```python
from build123d import *

# Parameters (mm, degrees)
SKETCH1_W           = 53.975
SKETCH1_H           = 31.75
BOSS_EXTRUDE1_DEPTH = 76.2
SHELL1_T            = 5
SKETCH2_W           = 44.45
SKETCH2_H           = 53.975
CUT_EXTRUDE1_DEPTH  = 5
FILLET1_R           = 31.75
FILLET2_R           = 6.35
FILLET3_R           = 6.35
SKETCH3_W           = 44.45
SKETCH3_H           = 53.975
BOSS_EXTRUDE2_DEPTH = 19.05
FILLET5_R           = 3.175
FILLET6_R           = 3.175


with BuildPart() as part:
    # Sketch1 → Boss-Extrude1 (new body)
    with BuildSketch(Plane(origin=(0, 0, 0), x_dir=(0, 0, -1), z_dir=(1, 0, 0))):
        with Locations((106.854663617, 0)):
            Rectangle(SKETCH1_W, SKETCH1_H)
    extrude(amount=BOSS_EXTRUDE1_DEPTH)

    # Shell1
    shell1_openings = [part.faces().sort_by_distance(p)[0] for p in [
        (0, 0, -106.854663617),
    ]]
    offset(amount=SHELL1_T, openings=shell1_openings, kind=Kind.INTERSECTION)

    # Sketch2 → Cut-Extrude1 (cut)
    with BuildSketch(Plane(origin=(0, -20.875, 0), x_dir=(-1, 0, 0), z_dir=(0, -1, 0))):
        with Locations((-53.975, 106.854663617)):
            Rectangle(SKETCH2_W, SKETCH2_H)
    extrude(amount=-CUT_EXTRUDE1_DEPTH, mode=Mode.SUBTRACT)

    # Fillet1
    fillet1_edges = [part.edges().sort_by_distance(p)[0] for p in [
        (76.2, 15.875, -106.854663617),
    ]]
    fillet(fillet1_edges, radius=FILLET1_R)

    # Fillet2
    # the kernel refuses this fillet: 6.35 mm, written as the material it takes off along each edge
    with BuildSketch(Plane(origin=(31.75, -15.875, -79.867163617), x_dir=(-1, 0, 0), z_dir=(0, 0, -1))) as fillet2_piece_1:
        with BuildLine():
            CenterArc((6.204836823, -6.35), FILLET2_R, 90, 77.725329785)
            Line((0, -5), (0, 0))
            Line((0, 0), (6.204836823, 0))
        make_face()
    extrude(amount=53.975, mode=Mode.SUBTRACT)

    # Fillet3
    fillet3_edges = [part.edges().sort_by_distance(p)[0] for p in [
        (81.2, 0, -138.842163617),
        (81.2, 20.875, -106.854663617),
        (81.2, 0, -74.867163617),
        (40.6, 20.875, -74.867163617),
        (40.6, 20.875, -138.842163617),
    ]]
    fillet(fillet3_edges, radius=FILLET3_R)

    # Sketch3 → Boss-Extrude2 (add)
    with BuildSketch(Plane.XZ.offset(20.875)):
        with BuildLine():
            Line((26.67, -74.867163617), (26.67, -138.842163617))
            Line((26.67, -138.842163617), (74.85, -138.842163617))
            ThreePointArc((74.85, -138.842163617), (79.340128061, -136.982291678), (81.2, -132.492163617))
            Line((81.2, -132.492163617), (81.2, -81.217163617))
            ThreePointArc((81.2, -81.217163617), (79.340128061, -76.727035557), (74.85, -74.867163617))
            Line((74.85, -74.867163617), (26.67, -74.867163617))
        make_face()
        with Locations((53.975, -106.854663617)):
            Rectangle(SKETCH3_W, SKETCH3_H, mode=Mode.SUBTRACT)
    extrude(amount=BOSS_EXTRUDE2_DEPTH)

    # Fillet5
    fillet5_edges = [part.edges().sort_by_distance(p)[0] for p in [
        (26.67, -20.875, -106.854663617),
    ]]
    fillet(fillet5_edges, radius=FILLET5_R)

    # Fillet6
    fillet6_edges = [part.edges().sort_by_distance(p)[0] for p in [
        (26.67, -39.925, -106.854663617),
        (50.76, -39.925, -138.842163617),
        (79.340128061, -39.925, -136.982291678),
        (81.2, -39.925, -106.854663617),
        (79.340128061, -39.925, -76.727035557),
        (50.76, -39.925, -74.867163617),
    ]]
    fillet(fillet6_edges, radius=FILLET6_R)


solid = part.part
```
Could you check a few things on this model? Use its own coordinates, in mm. A direction names the side the tool comes from. Coordinates: 2 decimals unless noted, no trailing zeros. Loops run counter-clockwise (first coordinate to the right, second up) from the corner with the lowest first, then second, coordinate; pieces in that order, holes last. Notation, with made-up numbers: M 85,18.5 L 127,18.5 A12 cw 127,34.5 Z; hole C -2.5,-30 d3. An arc over 180 degrees is marked long. Put each result on its own line as item: value. Start each with the question number.
(1) Suppose I cut it at C-C on z = -92. Please give me the cut outline in (x, y) (3 decimals).
(2) For faces 1 (the face through (26.67, -30, -106)), 2 (the face through (38, -12, -133.842)), 3 (the face through (76.2, -28, -107)), 4 (the face through (13, -15.875, -106)), which set-ups out of +Z, -Z, +X, -X, +Y, -Y let a thin tool reach every point of the face, with its end or its side?
(3) Suppose I cut it at A-A on y = -32. Please give me the cut outline in (x, z), then the cut area to 3 significant figures.
(4) Thinking about a two-plate mould opening in X: for faces 5 (the face through (36.9, 18.97, -76.68)), 6 (the face through (38, -12, -79.867)), 7 (the face through (66.652, 6.821, -107.232)), 8 (the face through (31.75, -30, -107)), which applies, pulls with the +X half, pulls with the -X half, needs draft (parallel to the pull), parting line crosses it, or undercut?
(5) Suppose I cut it at B-B on x = 16. Please give me the cut outline in (y, z) (3 decimals), then the cut area to 3 significant figures.
(6) Suppose I cut it at D-D on x = 40. Please give me the cut outline in (y, z) (3 decimals).
(7) I need wall thicknesses on line 1 (Z direction, x = 74, y = -29); line 2 (Y direction, x = 44, z = -98.5) (3 decimals); line 3 (Y direction, x = 17, z = -89) (3 decimals). Which ranges of each line are inside material? Lowest first, please. Write a range as from..to.
(8) Will these pins go through, and if not, where does the flat tip stop? P1, Ø11.5, axis at x = 10.5, z = -121, coming from the -Y side (3 decimals); P2, Ø6, axis at y = -8, z = -101.5, coming from the -X side; P3, Ø1, axis at y = -14.5, z = -111, coming from the -X side.
Solutions:
1. outline: M 0,-20.875 L 23.495,-20.875 A3.175 cw 26.67,-24.05 L 26.67,-36.75 A3.175 ccw 29.845,-39.925 L 31.75,-39.925 L 31.75,-20.875 A6.35 ccw 25.545,-15.875 L 0,-15.875 Z; M 0,15.875 L 44.45,15.875 A31.75 cw 76.2,-15.875 L 76.2,-39.925 L 78.025,-39.925 A3.175 ccw 81.2,-36.75 L 81.2,14.525 A6.35 ccw 74.85,20.875 L 0,20.875 Z
2. face 1: +Z, -Z, -X, -Y
2. face 2: none
2. face 3: -Y
2. face 4: -X
3. outline: M 26.67,-138.84 L 74.85,-138.84 A6.35 ccw 81.2,-132.49 L 81.2,-81.22 A6.35 ccw 74.85,-74.87 L 26.67,-74.87 Z; hole M 31.75,-133.84 L 76.2,-133.84 L 76.2,-79.87 L 31.75,-79.87 Z
3. area: 1,070 mm2
4. face 5: needs draft
4. face 6: undercut
4. face 7: pulls with the -X half
4. face 8: undercut
5. outline: M -20.875,-138.842 L 14.525,-138.842 A6.35 ccw 20.875,-132.492 L 20.875,-81.217 A6.35 ccw 14.525,-74.867 L -20.875,-74.867 Z; hole M -15.875,-133.842 L 15.875,-133.842 L 15.875,-79.867 L -15.875,-79.867 Z
5. area: 940 mm2
6. outline: M -39.925,-135.667 A3.175 ccw -36.75,-138.842 L 14.525,-138.842 A6.35 ccw 20.875,-132.492 L 20.875,-81.217 A6.35 ccw 14.525,-74.867 L -36.75,-74.867 A3.175 ccw -39.925,-78.042 L -39.925,-79.867 L 15.875,-79.867 L 15.875,-133.842 L -39.925,-133.842 Z
7. line 1: z = -138.84..-133.84, -79.87..-74.87
7. line 2: y = 15.875..20.875
7. line 3: y = -20.875..-15.875, 15.875..20.875
8. P1: stops at y = -20.875
8. P2: stops at x = 74.28
8. P3: stops at x = 76.14
